Could you check a few things on this model? Use its own coordinates, in mm. A direction names the side the tool comes from. Round coordinates to 2 decimals unless told otherwise and drop trailing zeros. Order: outer loops, then holes, each group sorted by start corner. A loop starts at its lowest first (then second) coordinate and runs counter-clockwise, first axis right, second up. Notation, with made-up numbers: (-4, 67.5) -> (32, 67.5) arc R13 cw to (32, 87.5) -> close; hole circle Ø3 at (-21, -6.75). An arc over 180 degrees is marked (long way). One line per question, with ' | ' between items.
```python
from build123d import *

# Parameters (mm, degrees)
BOSS_EXTRUDE1_DEPTH = 5
CUT_EXTRUDE1_DEPTH  = 5
SKETCH4_W           = 15.2
SKETCH4_H           = 5
CUT_EXTRUDE2_DEPTH  = 10


with BuildPart() as part:
    # Sketch1 → Boss-Extrude1 (new body)
    with BuildSketch(Plane.XY):
        Polygon((-22.5, 32.5), (0, 32.5), (22.5, 32.5), (22.5, -32.5), (-22.5, -32.5), (-22.5, -10), (-27.5, -10), (-27.5, 10), (-22.5, 10), align=None)
    extrude(amount=BOSS_EXTRUDE1_DEPTH)

    # Sketch3 → Cut-Extrude1 (cut)
    with BuildSketch(Plane.XY.offset(5)):
        Polygon((22.5, 24.5), (17.5, 24.5), (17.5, 26), (14.1, 26), (14.1, 24.5), (7.5, 24.5), (7.5, 20.1), (14.1, 20.1), (14.1, 18.6), (17.5, 18.6), (17.5, 20.1), (22.5, 20.1), align=None)
        Polygon((22.5, -24.5), (22.5, -20.1), (17.5, -20.1), (17.5, -18.6), (14.1, -18.6), (14.1, -20.1), (7.5, -20.1), (7.5, -24.5), (14.1, -24.5), (14.1, -26), (17.5, -26), (17.5, -24.5), align=None)
        Polygon((-22.5, -24.5), (-17.5, -24.5), (-17.5, -26), (-14.1, -26), (-14.1, -24.5), (-7.5, -24.5), (-7.5, -20.1), (-14.1, -20.1), (-14.1, -18.6), (-17.5, -18.6), (-17.5, -20.1), (-22.5, -20.1), align=None)
    extrude(amount=-CUT_EXTRUDE1_DEPTH, mode=Mode.SUBTRACT)

    # Sketch4 → Cut-Extrude2 (cut)
    with BuildSketch(Plane.XY.offset(5)):
        with Locations((0, -30)):
            Rectangle(SKETCH4_W, SKETCH4_H)
        with Locations((0, 30)):
            Rectangle(SKETCH4_W, SKETCH4_H)
    extrude(amount=-CUT_EXTRUDE2_DEPTH, mode=Mode.SUBTRACT)


solid = part.part
```
1. On a 3-axis mill with a long thin cutter (end or side, diameter ignored), from which of +Z, -Z, +X, -X, +Y, -Y can I reach the whole of each face in a straight line? I mean faces 1 (the face through (7.6, 30, 3)), 2 (the face through (11, -24.5, 3)), 3 (the face through (-16, -18.6, 3)), 4 (the face through (-7.5, -22, 3)), 5 (the face through (-22.5, -15, 2)). Say none if no direction works.
From the geometry:
face 1: +Z, -Z, +Y | face 2: +Z, -Z, +X | face 3: +Z, -Z | face 4: +Z, -Z, -X | face 5: +Z, -Z, -X, -Y
2. I want a section at B-B on x = -21. List the corners of the cut face in (y, z) for me, and give its area (3 significant figures).
From the geometry:
outline: (-32.5, 0) -> (-24.5, 0) -> (-24.5, 5) -> (-32.5, 5) -> close; (-20.1, 0) -> (32.5, 0) -> (32.5, 5) -> (-20.1, 5) -> close | area: 303 mm²
3. I want a section at C-C on y = -23. List the corners of the cut face in (x, z) for me, and give its area (3 significant figures).
From the geometry:
outline: (-7.5, 0) -> (7.5, 0) -> (7.5, 5) -> (-7.5, 5) -> close | area: 75.0 mm²
4. I'm going to push flat-ended pins straight in: pin 1 (0.8 mm diameter, centred on y = 19.5, z = 2.5, fed in from -X); pin 2 (1.5 mm diameter, centred on x = -26, z = 3.5, fed in from +Y). Where does each tip first touch, or does it pass through?
From the geometry:
pin 1: stops at x = -22.5 | pin 2: stops at y = 10
5. I need wall thicknesses on probe 1 along Y at (x, z) = (20, 0.8); probe 2 along Y at (x, z) = (14.5, 3.95); probe 3 along Y at (x, z) = (-13, 2.7). Which ranges of each line are inside material? Lowest first, please.
From the geometry:
probe 1: y = -32.5 to -24.5, -20.1 to 20.1, 24.5 to 32.5 | probe 2: y = -32.5 to -26, -18.6 to 18.6, 26 to 32.5 | probe 3: y = -32.5 to -24.5, -20.1 to 32.5
6. I want a section at A-A on x = 19. List the corners of the cut face in (y, z) for me.
From the geometry:
outline: (-32.5, 0) -> (-24.5, 0) -> (-24.5, 5) -> (-32.5, 5) -> close; (-20.1, 0) -> (20.1, 0) -> (20.1, 5) -> (-20.1, 5) -> close; (24.5, 0) -> (32.5, 0) -> (32.5, 5) -> (24.5, 5) -> close
7. I want a section at D-D on x = 1. List the corners of the cut face in (y, z) for me, and give its area (3 significant figures).
From the geometry:
outline: (-27.5, 0) -> (27.5, 0) -> (27.5, 5) -> (-27.5, 5) -> close | area: 275 mm²
8. If we mould it in two halves opening along Y, with no side actions, what happens to faces 6 (the face through (-27.5, 0, 2)), 7 (the face through (14.1, 19, 3)), 8 (the face through (-25, -10, 2))? For each: pulls with the +Y half, pulls with the -Y half, needs draft (parallel to the pull), parting line crosses it, or undercut.
From the geometry:
face 6: needs draft | face 7: undercut | face 8: pulls with the -Y half
